For this review, take the finished solid that the model builds, in its own axes (mm). A direction names the side the tool comes from. Round coordinates to 2 decimals unless told otherwise and drop trailing zeros. Write each loop counter-clockwise with the first axis right and the second up, starting at its lowest first coordinate (ties: lowest second). Pieces come first, ordered by that corner, then holes. Notation, with made-up numbers: (81.25, 78.25) -> (112.25, 78.25) arc R21 cw to (112.25, 91.25) -> close; hole circle Ø4 at (2, 58.5). An arc over 180 degrees is marked (long way). Write item = value, one per line. Start each with the question number.
```python
from build123d import *

# Parameters (mm, degrees)
SKETCH_208_R           = 4
SKETCH_208_R_2         = 1.5
SKETCH_208_R_3         = 2
EXTRUDE_1_DEPTH        = 2
SKETCH_3_R             = 2
EXTRUDE_2_DEPTH        = 2
SKETCH_4_W             = 20
SKETCH_4_H             = 22
SKETCH_4_R             = 1.5
EXTRUDE_3_DEPTH        = 2
FILLET_1_R             = 2
FILLET_1_OF_MIRROR_1_R = 2


with BuildPart() as part:
    # Sketch 208 → 凸台-拉伸1 (new body)
    with BuildSketch(Plane(origin=(0, 0, 0), x_dir=(1, 0, 0), z_dir=(0, 1, 0))):
        with BuildLine():
            Line((0, 36), (18, 36))
            Line((18, 36), (18, 26.5))
            Line((18, 26.5), (20, 26.5))
            Line((20, 26.5), (20, 32))
            Line((20, 32), (29, 32))
            Line((29, 32), (29, 8))
            Line((29, 8), (20, 8))
            Line((20, 8), (20, 0))
            Line((20, 0), (0, 0))
            Line((0, 0), (0, 5.5))
            ThreePointArc((0, 5.5), (1.5, 7), (0, 8.5))
            Line((0, 8.5), (0, 10))
            ThreePointArc((0, 10), (4, 14), (0, 18))
            Line((0, 18), (0, 19.5))
            ThreePointArc((0, 19.5), (1.5, 21), (0, 22.5))
            Line((0, 22.5), (0, 36))
        make_face()
        with Locations(Location((10, 24, 0), (0, 0, 270))):
            Circle(SKETCH_208_R, mode=Mode.SUBTRACT)
        with Locations(Location((10, 31, 0), (0, 0, 270))):
            Circle(SKETCH_208_R_2, mode=Mode.SUBTRACT)
        with Locations(Location((17, 24, 0), (0, 0, 270))):
            Circle(SKETCH_208_R_2, mode=Mode.SUBTRACT)
        with Locations(Location((10, 17, 0), (0, 0, 270))):
            Circle(SKETCH_208_R_2, mode=Mode.SUBTRACT)
        with Locations(Location((3, 24, 0), (0, 0, 270))):
            Circle(SKETCH_208_R_2, mode=Mode.SUBTRACT)
        with Locations(Location((7, 14, 0), (0, 0, 270))):
            Circle(SKETCH_208_R_2, mode=Mode.SUBTRACT)
        with Locations(Location((24, 24, 0), (0, 0, 270))):
            Circle(SKETCH_208_R_3, mode=Mode.SUBTRACT)
        with Locations(Location((24, 14, 0), (0, 0, 270))):
            Circle(SKETCH_208_R_3, mode=Mode.SUBTRACT)
    extrude_1 = extrude(amount=EXTRUDE_1_DEPTH)

    # 草图3 → 凸台-拉伸2 (add)
    with BuildSketch(Plane(origin=(0, 0, -32), x_dir=(-1, 0, 0), z_dir=(0, 0, -1))):
        Polygon((-20, 0), (-20, -23), (-29, -23), (-29, 0), (-29, 2), (-20, 2), align=None)
        with Locations((-24, -17)):
            Circle(SKETCH_3_R, mode=Mode.SUBTRACT)
        with Locations((-24, -7)):
            Circle(SKETCH_3_R, mode=Mode.SUBTRACT)
    extrude_2 = extrude(amount=-EXTRUDE_2_DEPTH)

    # 草图4 → 凸台-拉伸3 (add)
    with BuildSketch(Plane.XY):
        with Locations((10, -11)):
            Rectangle(SKETCH_4_W, SKETCH_4_H)
        with Locations((10, -10)):
            Circle(SKETCH_4_R, mode=Mode.SUBTRACT)
        with Locations((17, -10)):
            Circle(SKETCH_4_R, mode=Mode.SUBTRACT)
        with Locations((10, -17)):
            Circle(SKETCH_4_R, mode=Mode.SUBTRACT)
        with Locations((3, -10)):
            Circle(SKETCH_4_R, mode=Mode.SUBTRACT)
        with Locations((10, -3)):
            Circle(SKETCH_4_R, mode=Mode.SUBTRACT)
    extrude_3 = extrude(amount=-EXTRUDE_3_DEPTH)

    # 圆角1
    fillet_1_edges = [part.edges().sort_by_distance(p)[0] for p in [
        (20, -22, -1),
        (18, 1, -36),
        (29, 1, -8),
        (10, 2, 0),
        (24.5, 2, -32),
        (29, -23, -31),
        (20, -23, -31),
    ]]
    fillet(fillet_1_edges, radius=FILLET_1_R)

    # 镜向1: 凸台-拉伸1, 凸台-拉伸2, 凸台-拉伸3 across plane
    add(extrude_1.mirror(Plane(origin=(0, 0, 0), x_dir=(0, 0, 1), z_dir=(1, 0, 0))))
    add(extrude_2.mirror(Plane(origin=(0, 0, 0), x_dir=(0, 0, 1), z_dir=(1, 0, 0))))
    add(extrude_3.mirror(Plane(origin=(0, 0, 0), x_dir=(0, 0, 1), z_dir=(1, 0, 0))))

    # 圆角1 of 镜向1
    fillet_1_of_mirror_1_edges = [part.edges().sort_by_distance(p)[0] for p in [
        (-20, -22, -1),
        (-18, 1, -36),
        (-29, 1, -8),
        (-10, 2, 0),
        (-24.5, 2, -32),
        (-29, -23, -31),
        (-20, -23, -31),
    ]]
    fillet(fillet_1_of_mirror_1_edges, radius=FILLET_1_OF_MIRROR_1_R)


solid = part.part
```
1. Consider section B-B, the plane x = 10. Give the number of separate pieces and of enclosed holes in the cut face, then the cut area to 3 significant figures.
2. Consider section C-C, the plane y = -7. Give the boundary of the cut face in (x, z), then the cut area to 3 significant figures.
3. Machinability: for faces 4 (the cylindrical face through (-8.89, -1.99, -0.99)), 5 (the flat face through (-20, -7, -1)), which of the approach directions +Z, -Z, +X, -X, +Y, -Y give a long, thin tool a straight path to every point of the face, cutting with its end or side? Answer none if there is none.
4. Draft analysis for pull direction Y (two halves, no side actions). For faces 1 (the flat face through (19, 1, -26.5)), 2 (the cylindrical face through (-24, -15, -31)), 3 (the flat face through (0, -22, -1)), state which applies: +Y half, -Y half, draft (parallel to the pull), parting line (faces both ways), or undercut.
5. Wall thickness on L1, parallel to X at y = 1.5, z = -31; L2, parallel to X at y = 1.1, z = -14; L3, parallel to Y at x = -10, z = -1: over which ranges is each line inside the solid? List them lowest first. Write a range as from..to.
6. Consider section A-A, the plane z = -7. Give the boundary of the cut face in (x, y), then the cut area to 3 significant figures.
7. Clearance check with flat-ended pins moving along their axes: pin 1 Ø3 at (y, z) = (-6, -27.5) entering from +X; pin 2 Ø0.6 at (x, z) = (3, -0.5) entering from -Y; pin 3 Ø10 at (x, y) = (-24.5, -10) entering from -Z; pin 4 Ø5 at (x, y) = (3, -10) entering from +Z. State where each tip first meets the part, or that it passes through.
Outcome:
q1.separate_pieces = 7
q1.enclosed_holes = 0
q1.area = 69.1 mm2
q2.outline = (-29, -32) -> (-26, -32) -> (-26, -30) -> (-29, -30) -> close; (-22, -32) -> (-20, -32) -> (-20, -30) -> (-22, -30) -> close; (-20, -2) -> (20, -2) -> (20, 0) -> (-20, 0) -> close; (20, -32) -> (22, -32) -> (22, -30) -> (20, -30) -> close; (26, -32) -> (29, -32) -> (29, -30) -> (26, -30) -> close
q2.area = 100 mm2
q3.face_4 = +Z, -Z
q3.face_5 = +Z, -X, +Y, -Y
q4.face_1 = draft
q4.face_2 = undercut
q4.face_3 = -Y half
q5.L1 = -29..-20, -18..-11.5, -8.5..8.5, 11.5..18, 20..29
q5.L2 = -29..-26, -22..-8.5, -5.5..-4, 4..5.5, 8.5..22, 26..29
q5.L3 = -22..-18.5, -15.5..-11.5, -8.5..-4.5, -1.5..1.73
q6.outline = (-20, 0) -> (-1.5, 0) -> (-1.5, 2) -> (-20, 2) -> close; (1.5, 0) -> (20, 0) -> (20, 2) -> (1.5, 2) -> close
q6.area = 74.0 mm2
q7.pin_1 = through
q7.pin_2 = -22
q7.pin_3 = -32
q7.pin_4 = 0
